For this review, use the dimensioned drawing (mm, ordinates from the lowest corner) and the shaded views. Round coordinates to 2 decimals unless told otherwise and drop trailing zeros. Write each loop counter-clockwise with the first axis right and the second up, starting at its lowest first coordinate (ties: lowest second). Pieces come first, ordered by that corner, then holes. Notation, with made-up numbers: (-3, 68.25) - (22, 68.25) arc R19 ccw to (22, 91.25) - close; hole circle Ø9 at (-30, 1). An arc over 180 degrees is marked (long way). Return JSON: item names as keys, results as strings.
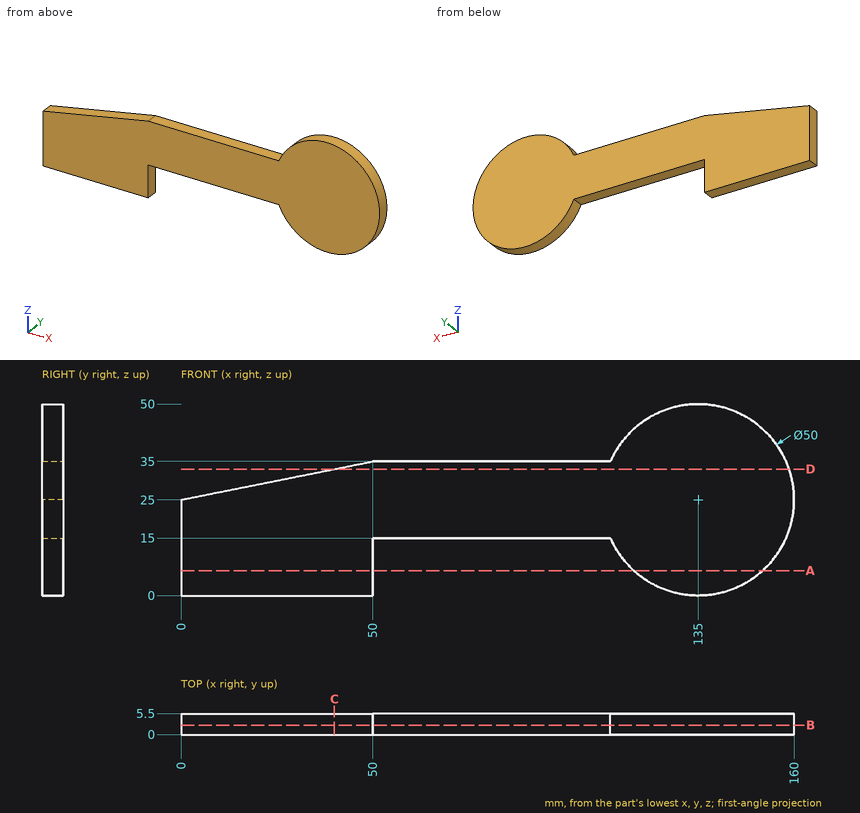
(1) Add section A-A (z = 6.5). Write out the cut boundary in (x, y).
Filled in:
{"outline": "(0, 0) - (50, 0) - (50, 5.5) - (0, 5.5) - close; (118.18, 0) - (151.82, 0) - (151.82, 5.5) - (118.18, 5.5) - close"}
(2) Wall thickness on line 1 (Z direction, x = 56, y = 4.2); line 2 (X direction, y = 1.1, z = 12); line 3 (X direction, y = 3.95, z = 9): over which ranges is each line inside the solid? List them lowest first.
Filled in:
{"line 1": "z = 15 to 35", "line 2": "x = 0 to 50, 113.65 to 156.35", "line 3": "x = 0 to 50, 115.79 to 154.21"}
(3) Add section D-D (z = 33). Write out the cut boundary in (x, y), plus the area to 3 significant figures.
Filled in:
{"outline": "(40, 0) - (158.69, 0) - (158.69, 5.5) - (40, 5.5) - close", "area": "653 mm2"}
(4) Add section B-B (y = 2.5). Write out the cut boundary in (x, z), plus the area to 3 significant figures.
Filled in:
{"outline": "(0, 0) - (50, 0) - (50, 15) - (112.09, 15) arc R25 ccw (long way) to (112.09, 35) - (50, 35) - (0, 25) - close", "area": "4,680 mm2"}
(5) Add section C-C (x = 40). Write out the cut boundary in (y, z), plus the area to 4 significant figures.
Filled in:
{"outline": "(0, 0) - (5.5, 0) - (5.5, 33) - (0, 33) - close", "area": "181.5 mm2"}
(6) Clearance check with flat-ended pins moving along their axes: pin 1 Ø1 at (x, y) = (57.5, 3) entering from +Z; pin 2 Ø1.5 at (y, z) = (4, 5.5) entering from +X; pin 3 Ø1.6 at (x, y) = (94, 2.5) entering from -Z. State where each tip first meets the part, or that it passes through.
Filled in:
{"pin 1": "stops at z = 35", "pin 2": "stops at x = 151.54", "pin 3": "stops at z = 15"}
